Autodesk Inventor part; units mm, degrees
ref_plane "YZ Plane" through (0, 0, 0) normal (1, 0, 0) x (0, 1, 0)
ref_plane "XZ Plane" through (0, 0, 0) normal (0, 1, 0) x (-1, 0, 0)
ref_plane "XY Plane" through (0, 0, 0) normal (0, 0, 1) x (1, 0, 0)
sketch "スケッチ1" plane through (0, 0, 0) normal (0, 1, 0) x (-1, 0, 0)
  circle A0 centre (0, 0) radius 6
  dimension "d0" = 12
extrude "押し出し1" add sketch "スケッチ1" along normal blind 40
sketch "スケッチ2" plane through (0, 40, 0) normal (0, 1, 0) x (1, 0, 0)
  point P0 (0, 0)
  point P1 (0, 0)
hole "穴1" at (0, 40, 0) direction (0, -1, 0) diameter 4.917 depth 12 tip angle 118
sketch "スケッチ3" plane through (0, 0, 0) normal (0, -1, 0) x (1, 0, 0)
  circle A0 centre (0, 0) radius 2.4585
hole "穴2" at (0, 0, 0) direction (0, 1, 0) diameter 4.917 depth 12 tip angle 118
properties part number "base_part5" material "アルミニウム 6061"
Build history of the part. All positions in model axes, mm. A direction names the side the tool comes from. Coordinates: 2 decimals unless noted, no trailing zeros. Write each loop counter-clockwise with the first axis right and the second up, starting at its lowest first coordinate (ties: lowest second). Pieces come first, ordered by that corner, then holes.
1. Drop flat-ended pins along their axis: pin 1 (1.5 mm diameter, centred on y = 6, z = -3, fed in from -X); pin 2 (1.5 mm diameter, centred on y = 28.5, z = -3, fed in from +X); pin 3 (5 mm diameter, centred on y = 21, z = 4.5, fed in from -X). Give the stop position or say it passes through.
Answer block:
pin 1: stops at x = -5.56
pin 2: stops at x = 5.56
pin 3: stops at x = -5.66
2. 3-axis set-ups, long thin cutter, end or side, ignore diameter. For faces 4 (the flat face through (-3, 0, 0)), 5 (the cylindrical face through (-0.738, 33.916, 2.345)): which of +Z, -Z, +X, -X, +Y, -Y reach the whole face in a straight line?
Answer block:
face 4: +Z, -Z, +X, -X, -Y
face 5: +Y
3. Band-saw the part on A-A, the plane y = 17. Give the cut face in (x, z).
Answer block:
outline: circle Ø12 at (0, 0)
4. Drill centre lines: probe 1 along Z at (x, y) = (0, 33.5); probe 2 along Z at (x, y) = (-1.75, 2); probe 3 along X at (y, z) = (6, 0.75). Where is each one in solid material? Low to high.
Answer block:
probe 1: z = -6 to -2.46, 2.46 to 6
probe 2: z = -5.74 to -1.73, 1.73 to 5.74
probe 3: x = -5.95 to -2.34, 2.34 to 5.95
5. Band-saw the part on B-B, the plane z = 5.25. Give the cut face in (x, y), and give its area (3 significant figures).
Answer block:
outline: (-2.9, 0) - (2.9, 0) - (2.9, 40) - (-2.9, 40) - close
area: 232 mm2
6. Pull direction Z, two halves, no side cores. Call faces 1 (the flat face through (-3, 40, 0)), 2 (the cylindrical face through (6, 20, 0)), 3 (the cylindrical face through (-0.738, 6.084, -2.345)): released by +Z, released by -Z, zero draft, split by the parting line, or undercut.
Answer block:
face 1: zero draft
face 2: split by the parting line
face 3: undercut
7. Band-saw the part on C-C, the plane x = -3.5. Give the cut face in (y, z).
Answer block:
outline: (0, -4.87) - (40, -4.87) - (40, 4.87) - (0, 4.87) - close
